Can you work these out from the model? Positions are in its coordinate system, mm. Round coordinates to 2 decimals unless told otherwise and drop trailing zeros. Write each loop counter-clockwise with the first axis right and the second up, starting at its lowest first coordinate (ties: lowest second). Pieces come first, ordered by that corner, then holes.
Q1. If we section it at D-D (x = 724): Please give me the cut outline in (y, z).
Q2. I'm going to push flat-ended pins straight in: pin 1 Ø1.5 at (x, z) = (-978.5, 18.5) entering from -Y; pin 2 Ø8 at (x, z) = (-480, -9) entering from +Y; pin 3 Ø10 at (y, z) = (44.5, 8) entering from +X. Where does each tip first touch, or does it pass through?
Q3. If we section it at C-C (y = -44): Give the number of separate pieces and of enclosed holes in the cut face, plus the area to 3 significant figures.
Q4. Please list where these lines run through material, in increasing order: line 1 along X through (y, z) = (2, -10); line 2 along Y through (x, z) = (1143, -17); line 3 along Y through (x, z) = (-1143, -16).
Q5. We'd pull the mould along X, two halves only. Please class faces 1 (the cylindrical face through (1244.576, 2.187, 0.533)), 2 (the flat face through (-1245, 1, 12.7)), 3 (the cylindrical face through (-1072.45, 54.09, -13.06)): +X half, -X half, draft (parallel to the pull), parting line (faces both ways), or undercut.
Q6. If we section it at A-A (x = -1164): Please give me the cut outline in (y, z).
Q7. If we section it at B-B (z = -15.5): Please give me the cut outline in (x, y), plus the area to 3 significant figures.
from build123d import *

# Parameters (mm, degrees)
SKETCH1_R               = 88.9
SKETCH1_R_2             = 76.2
BOSS_EXTRUDE1_DEPTH     = 38.1
CUT_EXTRUDE1_DEPTH      = 1364.467617688
CUT_EXTRUDE1_DEPTH_BACK = 1364.467617688
SKETCH2_W               = 304.8
SKETCH2_H               = 25.4
FILLET1_R               = 25.4


with BuildPart() as part:
    # Sketch1 → Boss-Extrude1 (new, symmetric)
    with BuildSketch(Plane.XY):
        with BuildLine():
            Line((-1137.073333333, 177.701194769), (1146.386666667, 101.543539868))
            ThreePointArc((1146.386666667, 101.543539868), (1244.6, 0), (1146.386666667, -101.543539868))
            Line((1146.386666667, -101.543539868), (-1137.073333333, -177.701194769))
            ThreePointArc((-1137.073333333, -177.701194769), (-1320.8, 0), (-1137.073333333, 177.701194769))
        make_face()
        with Locations(Location((-1143, 0, 0), (0, 0, 180))):
            Circle(SKETCH1_R, mode=Mode.SUBTRACT)
        with Locations(Location((1143, 0, 0), (0, 0, 180))):
            Circle(SKETCH1_R_2, mode=Mode.SUBTRACT)
    extrude(amount=BOSS_EXTRUDE1_DEPTH, both=True)

    # Sketch2 → Cut-Extrude1 (cut, two sides: drawn at the far end of the back side and taken through both)
    with BuildSketch(Plane(origin=(4.656666667, 139.622367318, 0), x_dir=(0.9994442900376634, -0.03333333333333318, 0), z_dir=(0.03333333333333318, 0.9994442900376634, 0)).offset(-CUT_EXTRUDE1_DEPTH_BACK)):
        with Locations((-1167.764823513, -25.4)):
            Rectangle(SKETCH2_W, SKETCH2_H)
    extrude(amount=CUT_EXTRUDE1_DEPTH + CUT_EXTRUDE1_DEPTH_BACK, mode=Mode.SUBTRACT)

    # Fillet1
    fillet1_edges = [part.edges().sort_by_distance(p)[0] for p in [
        (-1015.935828218, -0.193171338, 12.7),
    ]]
    fillet(fillet1_edges, radius=FILLET1_R - 0.0001)  # a hair under: the kernel refuses the full size


solid = part.part
A:
1. outline: (-115.63, -38.1) - (115.63, -38.1) - (115.63, 38.1) - (-115.63, 38.1) - close
2. pin 1: stops at y = -172.44
2. pin 2: stops at y = 155.92
2. pin 3: stops at x = 1236.61
3. separate pieces: 3
3. enclosed holes: 0
3. area: 170,000 mm2
4. line 1: x = -1320.79 to -1231.88, -1054.12 to 1066.83, 1219.17 to 1244.58
4. line 2: y = -101.66 to -76.2, 76.2 to 101.66
4. line 3: y = -177.8 to -88.9, 88.9 to 177.8
5. face 1: +X half
5. face 2: draft
5. face 3: undercut
6. outline: (-176.56, -38.1) - (-86.38, -38.1) - (-86.38, 12.7) - (-176.56, 12.7) - close; (86.38, -38.1) - (176.56, -38.1) - (176.56, 12.7) - (86.38, 12.7) - close
7. outline: (-1137.07, -177.7) - (1146.39, -101.54) arc R101.6 ccw to (1146.39, 101.54) - (-1137.07, 177.7) arc R177.8 ccw (long way) to start; hole circle Ø177.8 at (-1143, 0); hole circle Ø152.4 at (1143, 0)
7. area: 662,000 mm2
